Part model, mm, in its own coordinate system. Face numbers are marked on the shaded views. A direction names the side the tool comes from. Round coordinates to 2 decimals unless told otherwise and drop trailing zeros. Order: outer loops, then holes, each group sorted by start corner. A loop starts at its lowest first (then second) coordinate and runs counter-clockwise, first axis right, second up. Notation, with made-up numbers: (70, 83) -> (98, 83) arc R19 cw to (98, 111) -> close; hole circle Ø3 at (84.25, 76.5). An arc over 180 degrees is marked (long way). Answer as a JSON object with one key per item and string values. Group by question number.
```python
from build123d import *

# Parameters (mm, degrees)
F1_DEPTH  = 63.5
F2_DEPTH  = 25.4
F3_DEPTH  = 7.9375
F2_FACE_W = 50.8
F2_FACE_H = 19.05
F4_DEPTH  = 25.4
F6_R      = 5.08


with BuildPart() as f1:
    # F0 (on Front) → F1 (new body, symmetric)
    with BuildSketch(Plane.XZ):
        Polygon((22.225, 9.525), (-41.275, 9.525), (-41.275, -9.525), (41.275, -9.525), (41.275, 9.525), align=None)
    extrude(amount=F1_DEPTH, both=True)

    # F0 (on Front) → F2 (join, symmetric)
    with BuildSketch(Plane.XZ):
        with BuildLine():
            Line((22.225, 27.0002), (22.225, 9.525))
            Line((22.225, 9.525), (41.275, 9.525))
            Line((41.275, 9.525), (41.275, 27.0002))
            ThreePointArc((41.275, 27.0002), (45.92468, 38.22552), (57.15, 42.8752))
            Line((57.15, 42.8752), (60.325, 42.8752))
            Line((60.325, 42.8752), (60.325, 61.9252))
            Line((60.325, 61.9252), (57.15, 61.9252))
            add(Edge.make_bspline(
                [(54.567041, 61.829555), (55.435808, 61.866108), (56.29704, 61.897928), (57.15, 61.9252)],
                knots=[109.116845, 109.116845, 109.116845, 109.116845, 111.504536, 111.504536, 111.504536, 111.504536], degree=3))
            ThreePointArc((54.567041, 61.829555), (31.557369, 50.765151), (22.225, 27.0002))
        make_face()
    extrude(amount=F2_DEPTH, both=True)

    # F0 (on Front) → F3 (join, symmetric)
    with BuildSketch(Plane.XZ):
        with BuildLine():
            add(Edge.make_bspline(
                [(-41.275, 9.525), (-40.572758, 48.603796), (14.864627, 60.159082), (54.567041, 61.829555)],
                knots=[0, 0, 0, 0, 109.116845, 109.116845, 109.116845, 109.116845], degree=3))
            Line((-41.275, 9.525), (22.225, 9.525))
            Line((22.225, 9.525), (22.225, 27.0002))
            ThreePointArc((22.225, 27.0002), (31.557369, 50.765151), (54.567041, 61.829555))
        make_face()
    extrude(amount=F3_DEPTH, both=True)

    # F2_face (on face) → F4 (join)
    with BuildSketch(Plane(origin=(60.325, 0, 52.4002), x_dir=(0, 1, 0), z_dir=(1, 0, 0))):
        Rectangle(F2_FACE_W, F2_FACE_H)
    extrude(amount=F4_DEPTH)

    # F0 (on Front) → F5 (revolve)
    with BuildSketch(Plane.XZ):
        Polygon((80.682018, 66.675), (80.682018, 61.9252), (80.682018, 42.8752), (80.682018, 38.1), (111.125, 38.1), (111.125, 66.675), align=None)
    revolve(axis=Axis((80.682018, 0, 52.3875), (0, 0, 1)))

    # F6
    f6_edges = [f1.edges().sort_by_distance(p)[0] for p in [
        (-41.275, 63.5, 0),
        (-41.275, -63.5, 0),
        (41.275, 63.5, 0),
        (41.275, -63.5, 0),
    ]]
    fillet(f6_edges, radius=F6_R)


solid = f1.part
```
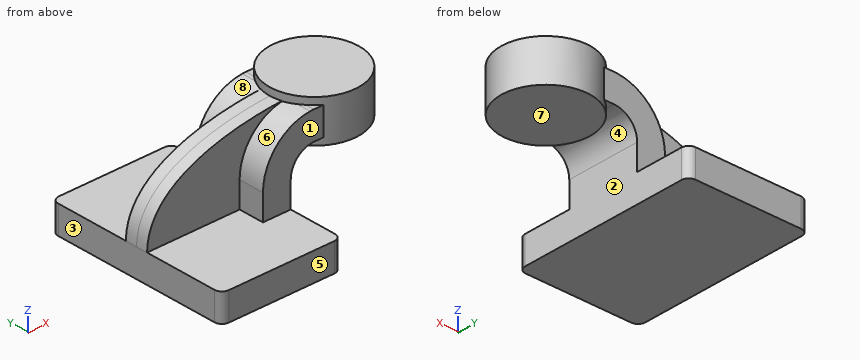
Q1. Drop flat-ended pins along their axis: pin 1 Ø21 at (x, z) = (34.5, 36.5) entering from -Y; pin 2 Ø18.5 at (x, y) = (77, -7.5) entering from -Z; pin 3 Ø6 at (x, z) = (27, 32) entering from +Y. Give the stop position or say it passes through.
Q2. Wall check: line 1 (Z direction, x = 75, y = -14.5) (3 decimals); line 2 (Y direction, x = 30.5, z = 52.5); line 3 (Z direction, x = -22, y = 8) (3 decimals). Give the ranges that are in metal, low to high. Write a range as [from, to].
Q3. Which spindle directions (+Z, -Z, +X, -X, +Y, -Y) get a long thin tool onto all of the face, cutting with end or side? Do the marked faces 5, 6, 7 and 8. Say none if no direction does.
Q4. Two-plate mould, pull along X, no slides. Class the marked faces 1, 2, 3 and 4: +X half, -X half, draft (parallel to the pull), parting line (faces both ways), or undercut.
Q5. Band-saw the part on D-D (x = 90). List the corners of the cut face in (y, z) (3 decimals).
Q6. Band-saw the part on A-A (z = 6). List the corners of the cut face in (x, y) (3 decimals), plus the area to 3 significant figures.
Q7. Band-saw the part on B-B (x = 59.5). List the corners of the cut face in (y, z) (3 decimals).
Q8. Band-saw the part on C-C (y = -39). List the corners of the cut face in (x, z) (3 decimals).
Completed:
{
 "1": {"pin 1": "y = -25.4", "pin 2": "z = 38.1", "pin 3": "y = 25.4"},
 "2": {"line 1": "[38.1, 66.675]", "line 2": "[-7.94, 7.94]", "line 3": "[-9.525, 9.525]"},
 "3": {"face 5": "+Z, -Z, +X, -X, -Y", "face 6": "+Z, -X, -Y", "face 7": "-Z, +X, +Y, -Y", "face 8": "+Z, -X, +Y"},
 "4": {"face 1": "draft", "face 2": "+X half", "face 3": "-X half", "face 4": "undercut"},
 "5": {"outline": "(-28.982, 38.1) -> (28.982, 38.1) -> (28.982, 66.675) -> (-28.982, 66.675) -> close"},
 "6": {"outline": "(-41.275, -58.42) arc R5.08 ccw to (-36.195, -63.5) -> (36.195, -63.5) arc R5.08 ccw to (41.275, -58.42) -> (41.275, 58.42) arc R5.08 ccw to (36.195, 63.5) -> (-36.195, 63.5) arc R5.08 ccw to (-41.275, 58.42) -> close", "area": "10,500 mm2"},
 "7": {"outline": "(-25.4, 42.875) -> (-21.865, 42.875) -> (-21.865, 38.1) -> (21.865, 38.1) -> (21.865, 42.875) -> (25.4, 42.875) -> (25.4, 61.925) -> (21.865, 61.925) -> (21.865, 66.675) -> (-21.865, 66.675) -> (-21.865, 61.925) -> (-25.4, 61.925) -> close"},
 "8": {"outline": "(-41.275, -9.525) -> (41.275, -9.525) -> (41.275, 9.525) -> (-41.275, 9.525) -> close"}
}
